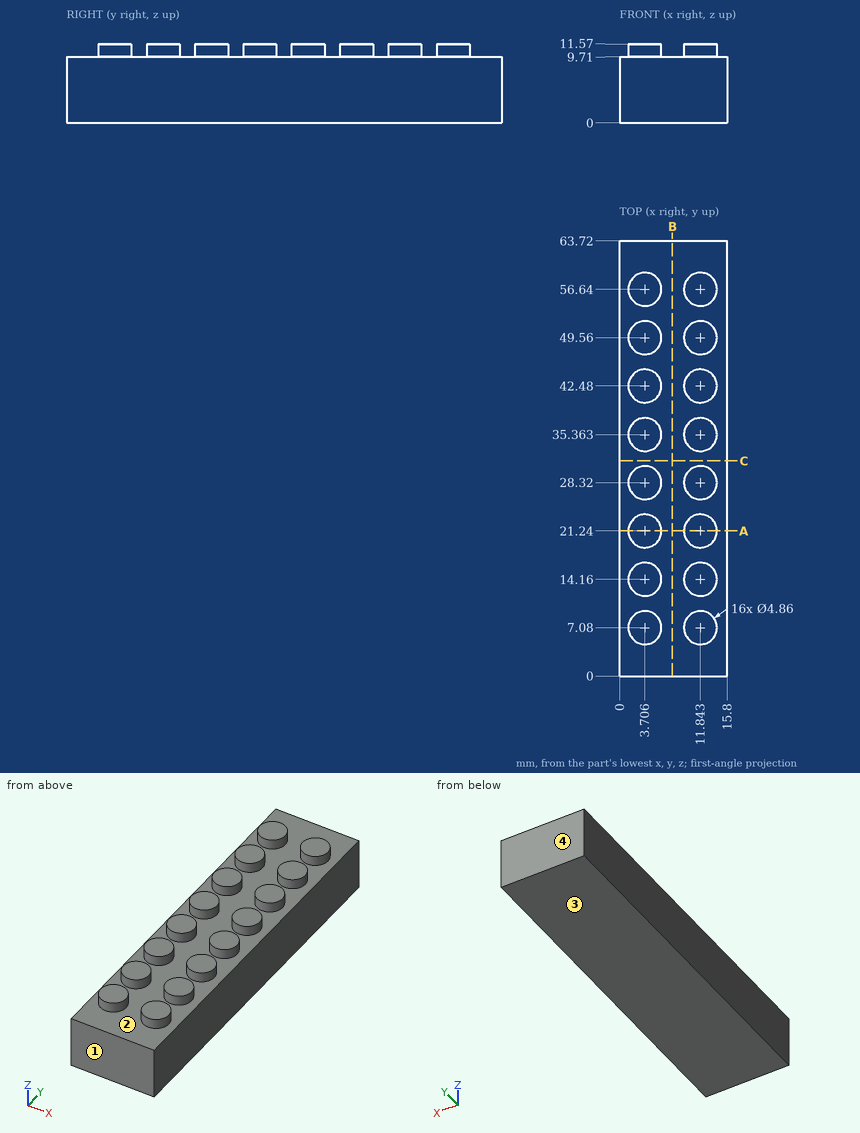
Could you check a few things on this drawing? It's one solid part, dimensions in mm from its lowest x, y, z. Give positions to 0.01 mm unless a question says otherwise; leave off trailing zeros. Order: outer loops, then holes, each group sorted by start corner. A loop starts at its lowest first (then second) coordinate and runs counter-clockwise, first axis right, second up. Notation, with made-up numbers: (-1, -10.5) - (18, -10.5) arc R21 cw to (18, 25.5) - close; hole circle Ø3 at (1, 28.25). An arc over 180 degrees is marked (long way). One line per question, with ' | ' between items. Start each with the question number.
Item 1: I need wall thicknesses on probe 1 along Z at (x, y) = (9.5, 60.5); probe 2 along X at (y, z) = (36, 10.5); probe 3 along X at (y, z) = (13, 10). Which ranges of each line are inside material? Lowest first, please. Write a range as [from, to].
Item 2: Thinking about a two-plate mould opening in Y: for the marked faces 1, 2, 3 and 4, which applies, pulls with the +Y half, pulls with the -Y half, needs draft (parallel to the pull), parting line crosses it, or undercut?
Item 3: I want a section at B-B on x = 7.75. Write out the boundary of the cut face in (y, z).
Item 4: I want a section at A-A on y = 21.24. Write out the boundary of the cut face in (x, z) (1 decimal).
Item 5: I want a section at C-C on y = 31.5. Write out the boundary of the cut face in (x, z).
Item 6: I'm going to push a flat-ended pin straight in: pin 1 Ø8 at (x, y) = (3, 37.5) entering from -Z. Where does the tip first touch, or does it pass through?
Verdict:
1) probe 1: [0, 9.71] | probe 2: [1.36, 6.05], [9.5, 14.19] | probe 3: [1.57, 5.84], [9.71, 13.98]
2) face 1: pulls with the -Y half | face 2: undercut | face 3: needs draft | face 4: pulls with the +Y half
3) outline: (0, 0) - (63.72, 0) - (63.72, 9.71) - (0, 9.71) - close
4) outline: (0, 0) - (15.8, 0) - (15.8, 9.7) - (14.3, 9.7) - (14.3, 11.6) - (9.4, 11.6) - (9.4, 9.7) - (6.1, 9.7) - (6.1, 11.6) - (1.3, 11.6) - (1.3, 9.7) - (0, 9.7) - close
5) outline: (0, 0) - (15.8, 0) - (15.8, 9.71) - (0, 9.71) - close
6) pin 1: z = 0
